The drawing under review shows one solid part. Ordinate dimensions are in mm from its lowest x, y, z. Coordinates: 2 decimals unless noted, no trailing zeros. Loops run counter-clockwise (first coordinate to the right, second up) from the corner with the lowest first, then second, coordinate; pieces in that order, holes last. Notation, with made-up numbers: M 50,76 L 63,76 A36 cw 63,110 Z; hole C 25,45.5 d2. An arc over 180 degrees is marked long. Return JSON: item names as keys, results as strings.
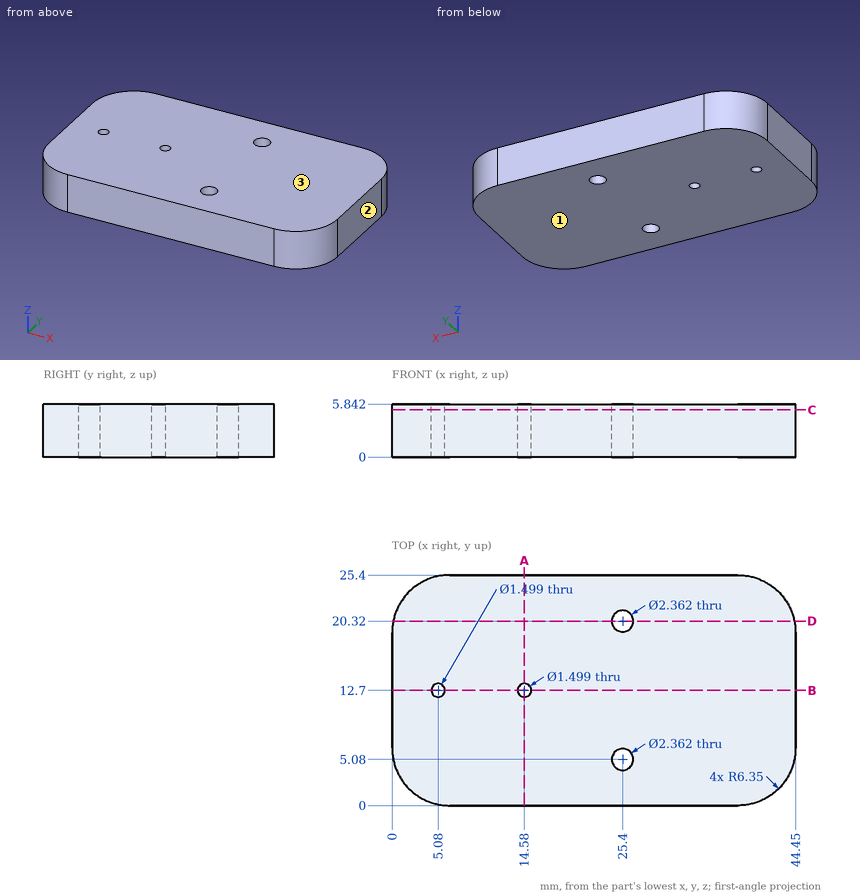
1. To check wall thickness, follow line 1 (Y direction, x = 25.4, z = 3.35); line 2 (X direction, y = 12.7, z = 3.45); line 3 (Y direction, x = 14.58, z = 3.4). State the ranges of each line that lie inside material, in increasing order.
Check values:
{"line 1": "0 to 3.9, 6.26 to 19.14, 21.5 to 25.4", "line 2": "0 to 4.33, 5.83 to 13.83, 15.33 to 44.45", "line 3": "0 to 11.95, 13.45 to 25.4"}
2. Add section A-A on x = 14.58. Give the boundary of the cut face in (y, z).
Check values:
{"outline": "M 0,0 L 11.95,0 L 11.95,5.84 L 0,5.84 Z; M 13.45,0 L 25.4,0 L 25.4,5.84 L 13.45,5.84 Z"}
3. Insertion check: pin 1 Ø3 at (y, z) = (21, 2) entering from -X. The pin has a flat end and moves straight along its axis. Give the tip position at first contact, or say it passes through.
Check values:
{"pin 1": "x = 0.02"}
4. Add section B-B on y = 12.7. Give the boundary of the cut face in (x, z).
Check values:
{"outline": "M 0,0 L 4.33,0 L 4.33,5.84 L 0,5.84 Z; M 5.83,0 L 13.83,0 L 13.83,5.84 L 5.83,5.84 Z; M 15.33,0 L 44.45,0 L 44.45,5.84 L 15.33,5.84 Z"}
5. Add section D-D on y = 20.32. Give the boundary of the cut face in (x, z).
Check values:
{"outline": "M 0.13,0 L 24.22,0 L 24.22,5.84 L 0.13,5.84 Z; M 26.58,0 L 44.32,0 L 44.32,5.84 L 26.58,5.84 Z"}
6. The part is to be moulded in two halves that separate along Z. For the marked faces 1, 2 and 3, say which applies: released by +Z, released by -Z, zero draft, split by the parting line, or undercut.
Check values:
{"face 1": "released by -Z", "face 2": "zero draft", "face 3": "released by +Z"}
7. Add section C-C on z = 5.2. Give the boundary of the cut face in (x, y), plus the area to 3 significant figures.
Check values:
{"outline": "M 0,6.35 A6.35 ccw 6.35,0 L 38.1,0 A6.35 ccw 44.45,6.35 L 44.45,19.05 A6.35 ccw 38.1,25.4 L 6.35,25.4 A6.35 ccw 0,19.05 Z; hole C 5.08,12.7 d1.5; hole C 14.58,12.7 d1.5; hole C 25.4,5.08 d2.36; hole C 25.4,20.32 d2.36", "area": "1,080 mm²"}
